Verification items for the finished model (mm, model axes). A direction names the side the tool comes from. Round coordinates to 2 decimals unless told otherwise and drop trailing zeros. Order: outer loops, then holes, each group sorted by start corner. A loop starts at its lowest first (then second) coordinate and runs counter-clockwise, first axis right, second up. Notation, with made-up numbers: M 37.25,27 L 45.25,27 A8 ccw 45.25,32 Z; hole C -27.75,63.5 d5. An arc over 180 degrees is marked long. One line per item, written item: value. Start each with the question number.
from build123d import *

# Parameters (mm, degrees)
ESQUISSE1_W             = 63.5
ESQUISSE1_H             = 24.82
ESQUISSE1_R             = 6
BOSS_EXTRU_1_DEPTH      = 6
ESQUISSE2_R             = 1.5
ENL_V_MAT_EXTRU_1_DEPTH = 10
ESQUISSE3_R             = 1.5
ENL_V_MAT_EXTRU_2_DEPTH = 10


with BuildPart() as part:
    # Esquisse1 → Boss.-Extru.1 (new body)
    with BuildSketch(Plane.XY):
        with Locations((13.304900678, -1.402259887)):
            Rectangle(ESQUISSE1_W, ESQUISSE1_H)
        with Locations((3.554900678, -1.402259887)):
            Circle(ESQUISSE1_R, mode=Mode.SUBTRACT)
    extrude(amount=BOSS_EXTRU_1_DEPTH)

    # Esquisse2 → Enlèv. mat.-Extru.1 (cut)
    with BuildSketch(Plane(origin=(45.054900678, 0, 0), x_dir=(0, 0, -1), z_dir=(1, 0, 0))):
        with Locations((-3, 7.597740113)):
            Circle(ESQUISSE2_R)
        with Locations((-3, -10.402259887)):
            Circle(ESQUISSE2_R)
    extrude(amount=-ENL_V_MAT_EXTRU_1_DEPTH, mode=Mode.SUBTRACT)

    # Esquisse3 → Enlèv. mat.-Extru.2 (cut)
    with BuildSketch(Plane(origin=(0, 0, 0), x_dir=(-1, 0, 0), z_dir=(0, 0, -1))):
        with Locations((14.031893584, 7.597740113)):
            Circle(ESQUISSE3_R)
        with Locations((14.031893584, -10.402259887)):
            Circle(ESQUISSE3_R)
    extrude(amount=-ENL_V_MAT_EXTRU_2_DEPTH, mode=Mode.SUBTRACT)


solid = part.part
1. Section check C-C (y = -9.75). Record the cut outline in (x, z), and give its area (3 significant figures).
2. Depth check by flat-ended pin: pin 1 (2.5 mm diameter, centred on y = 7.6, z = 3, fed in from +X). Enter the tip coordinate at first touch or a pass-through.
3. Section check D-D (x = 40). Record the cut outline in (y, z), and give its area (3 significant figures).
4. Scan lines: line 1 along Y through (x, z) = (38.5, 3); line 2 along Y through (x, z) = (40.5, 3.7); line 3 along X through (y, z) = (-11.75, 4.35). Record each from-to range of solid material in increasing order.
5. Tool access check on faces 5 (the face through (35.055, 8, 3)), 6 (the face through (13, -1, 6)). Record the directions out of +Z, -Z, +X, -X, +Y, -Y that give a thin tool (end or side, any length) a straight path to the whole face; none if there is none.
6. Section check B-B (z = 3). Record the cut outline in (x, y).
7. Draft check along Z on faces 1 (the face through (13, -1, 0)), 2 (the face through (13, 11.008, 3)), 3 (the face through (40.125, -11.733, 2.308)), 4 (the face through (35.055, -10, 3)). Enter one of: released by +Z, released by -Z, zero draft, split by the parting line, or undercut.
8. Section check A-A (x = 7). Record the cut outline in (y, z).
Geometry check:
1. outline: M -18.45,0 L -15.38,0 L -15.38,6 L -18.45,6 Z; M -12.68,0 L 45.05,0 L 45.05,1.65 L 35.05,1.65 L 35.05,4.35 L 45.05,4.35 L 45.05,6 L -12.68,6 Z
1. area: 338 mm²
2. pin 1: stops at x = 35.05
3. outline: M -13.81,0 L 11.01,0 L 11.01,6 L -13.81,6 Z; hole C -10.4,3 d3; hole C 7.6,3 d3
3. area: 135 mm²
4. line 1: y = -13.81 to -11.9, -8.9 to 6.1, 9.1 to 11.01
4. line 2: y = -13.81 to -11.73, -9.08 to 6.27, 8.92 to 11.01
4. line 3: x = -18.45 to -14.69, -13.37 to 45.05
5. face 5: +X
5. face 6: +Z, +X, -X, +Y, -Y
6. outline: M -18.45,-13.81 L 45.05,-13.81 L 45.05,-11.9 L 35.05,-11.9 L 35.05,-8.9 L 45.05,-8.9 L 45.05,6.1 L 35.05,6.1 L 35.05,9.1 L 45.05,9.1 L 45.05,11.01 L -18.45,11.01 Z; hole C -14.03,-10.4 d3; hole C -14.03,7.6 d3; hole C 3.55,-1.4 d12
7. face 1: released by -Z
7. face 2: zero draft
7. face 3: undercut
7. face 4: undercut
8. outline: M -13.81,0 L -6.31,0 L -6.31,6 L -13.81,6 Z; M 3.51,0 L 11.01,0 L 11.01,6 L 3.51,6 Z
